Work out the finished part from the listing and answer in its coordinate system (mm). A direction names the side the tool comes from. Give positions to 0.01 mm unless a question says otherwise; leave off trailing zeros. Write each loop counter-clockwise with the first axis right and the second up, starting at its lowest first coordinate (ties: lowest second). Pieces come first, ordered by that corner, then holes.
1) Find section D-D (y = 5.75). Determine the outline of the cut face in (x, z), plus the area to 3 significant figures.
2) Given pin 1 Ø1.5 at (x, z) = (0, -2.5) entering from +Y; pin 2 Ø1.1 at (y, z) = (2.5, -8) entering from -X; pin 3 Ø1.1 at (y, z) = (-0.5, -8) entering from +X, each flat-ended and moving along its own axis, determine where each tip first touches the part or whether it passes through.
3) A tool of negligible diameter and unlimited length cuts with its end or side. For faces 1 (the face through (-10.43, 0.11, -6.45)), 2 (the face through (-25.359, 0.105, -8.797)), 3 (the face through (10.43, -0.11, -9.55)), from which of +Z, -Z, +X, -X, +Y, -Y can it reach the whole face along a straight path? Write none if from no direction.
4) Determine the mould class of faces 4 (the face through (22.07, -0.11, -5.55)), 5 (the face through (26.5, 0, 0)), 6 (the face through (-10.43, 0.11, -9.55)), 7 (the face through (0, 3, 6)) for opening direction Z: pulls with the +Z half, pulls with the -Z half, needs draft (parallel to the pull), parting line crosses it, or undercut.
5) Find section A-A (x = 0). Determine the outline of the cut face in (y, z).
6) Straight lines are drawn through the part: probe 1 along Z at (x, y) = (17.5, -3); probe 2 along Y at (x, z) = (0, 5.1); probe 3 along X at (y, z) = (4.75, -2.5). For each, find the intervals that lie inside material, in ascending order.
7) Find section B-B (y = 0). Determine the outline of the cut face in (x, z).
8) Find section C-C (z = 3.5). Determine the outline of the cut face in (x, y), plus the area to 3 significant figures.
```python
from build123d import *

# Parameters (mm, degrees)
EXTRU_MINCE1_DEPTH                             = 7.5
ESQUISSE4_W                                    = 53
ESQUISSE4_H                                    = 15
BOSS_EXTRU_1_DEPTH                             = 2
FRAISAGE_POUR_VIS_T_TE_FRAIS_E_M41_D           = 4
FRAISAGE_POUR_VIS_T_TE_FRAIS_E_M41_CSINK_D     = 8
FRAISAGE_POUR_VIS_T_TE_FRAIS_E_M41_CSINK_ANGLE = 90
CONG_1_R                                       = 1.5
CONG_2_R                                       = 4


with BuildPart() as part:
    # Esquisse1 → Extru.-Mince1 (new, symmetric)
    with BuildSketch(Plane(origin=(0, 0, 0), x_dir=(1, 0, 0), z_dir=(0, 1, 0))):
        Polygon((-10, 6), (-22.5, 6), (-22.5, 0), (22.5, 0), (22.5, 6), (10, 6), (10, 10), (26.5, 10), (26.5, -4), (-26.5, -4), (-26.5, 10), (-10, 10), align=None)
    extrude(amount=EXTRU_MINCE1_DEPTH, both=True)

    # Esquisse4 → Boss.-Extru.1 (add)
    with BuildSketch(Plane.XY.offset(4)):
        Rectangle(ESQUISSE4_W, ESQUISSE4_H)
    extrude(amount=BOSS_EXTRU_1_DEPTH)

    # Fraisage pour vis à tête fraisée M41 (through all)
    with Locations(Plane(origin=(0, 0, 0), x_dir=(-1, 0, 0), z_dir=(0, 0, -1))):
        with Locations((0, 0)):
            CounterSinkHole(FRAISAGE_POUR_VIS_T_TE_FRAIS_E_M41_D / 2, FRAISAGE_POUR_VIS_T_TE_FRAIS_E_M41_CSINK_D / 2, counter_sink_angle=FRAISAGE_POUR_VIS_T_TE_FRAIS_E_M41_CSINK_ANGLE)

    # Congé1
    cong_1_edges = [part.edges().sort_by_distance(p)[0] for p in [
        (-22.5, 0, -6),
        (-22.5, 0, 0),
        (22.5, 0, 0),
        (22.5, 0, -6),
        (10, 0, -6),
        (10, 0, -10),
        (-10, 0, -10),
        (-10, 0, -6),
    ]]
    fillet(cong_1_edges, radius=CONG_1_R)

    # Congé2
    cong_2_edges = [part.edges().sort_by_distance(p)[0] for p in [
        (26.5, 0, -10),
        (-26.5, 0, -10),
    ]]
    fillet(cong_2_edges, radius=CONG_2_R)


solid = part.part
```
Results:
1. outline: (-26.5, -6) arc R4 ccw to (-22.5, -10) - (-11.5, -10) arc R1.5 ccw to (-10, -8.5) - (-10, -7.5) arc R1.5 ccw to (-11.5, -6) - (-21, -6) arc R1.5 cw to (-22.5, -4.5) - (-22.5, -1.5) arc R1.5 cw to (-21, 0) - (21, 0) arc R1.5 cw to (22.5, -1.5) - (22.5, -4.5) arc R1.5 cw to (21, -6) - (11.5, -6) arc R1.5 ccw to (10, -7.5) - (10, -8.5) arc R1.5 ccw to (11.5, -10) - (22.5, -10) arc R4 ccw to (26.5, -6) - (26.5, 6) - (-26.5, 6) - close
1. area: 491 mm2
2. pin 1: passes through
2. pin 2: stops at x = -26.23
2. pin 3: stops at x = 26.23
3. face 1: +Y, -Y
3. face 2: -Z, -X, +Y, -Y
3. face 3: -Z, +Y, -Y
4. face 4: undercut
4. face 5: needs draft
4. face 6: pulls with the -Z half
4. face 7: pulls with the +Z half
5. outline: (-7.5, 0) - (-4, 0) - (-2, 2) - (-2, 6) - (-7.5, 6) - close; (2, 2) - (4, 0) - (7.5, 0) - (7.5, 6) - (2, 6) - close
6. probe 1: z = -10 to -6, 0 to 6
6. probe 2: y = -7.5 to -2, 2 to 7.5
6. probe 3: x = -26.5 to -22.5, 22.5 to 26.5
7. outline: (-26.5, -6) arc R4 ccw to (-22.5, -10) - (-11.5, -10) arc R1.5 ccw to (-10, -8.5) - (-10, -7.5) arc R1.5 ccw to (-11.5, -6) - (-21, -6) arc R1.5 cw to (-22.5, -4.5) - (-22.5, -1.5) arc R1.5 cw to (-21, 0) - (-4, 0) - (-2, 2) - (-2, 6) - (-26.5, 6) - close; (2, 2) - (4, 0) - (21, 0) arc R1.5 cw to (22.5, -1.5) - (22.5, -4.5) arc R1.5 cw to (21, -6) - (11.5, -6) arc R1.5 ccw to (10, -7.5) - (10, -8.5) arc R1.5 ccw to (11.5, -10) - (22.5, -10) arc R4 ccw to (26.5, -6) - (26.5, 6) - (2, 6) - close
8. outline: (-26.5, -7.5) - (26.5, -7.5) - (26.5, 7.5) - (-26.5, 7.5) - close; hole circle Ø4 at (0, 0)
8. area: 782 mm2
